from build123d import *

# Parameters (mm, degrees)
SKETCH1_W                     = 113.95
SKETCH1_H                     = 50
BOSS_EXTRUDE1_DEPTH           = 2
SKETCH2_W                     = 8
SKETCH2_H                     = 50
BOSS_EXTRUDE2_DEPTH           = 3
SKETCH3_W                     = 2
SKETCH3_H                     = 50
BOSS_EXTRUDE3_DEPTH           = 4
SKETCH7_W                     = 6
SKETCH7_H                     = 8
BOSS_EXTRUDE5_DEPTH           = 8
FILLET1_RADIUS                = 3
FILLET1_LENGTH                = 8
SKETCH10_R                    = 1.525
CUT_EXTRUDE2_DEPTH            = 2
LPATTERN2_COUNT               = 2
LPATTERN2_PITCH               = 20
FILLET1_OF_LPATTERN2_2_RADIUS = 3
FILLET1_OF_LPATTERN2_2_LENGTH = 8
FILLET2_R                     = 3
FILLET3_R                     = 3
FILLET4_START                 = -25
FILLET4_DEPTH                 = 20
FILLET4_START_2               = 3
FILLET4_2_DEPTH               = 12
FILLET4_START_3               = -19.719
FILLET4_3_DEPTH               = 44.719
FILLET4_START_4               = 23
FILLET4_4_DEPTH               = 2
FILLET5_R                     = 3


with BuildPart() as part:
    # Sketch1 → Boss-Extrude1 (new body)
    with BuildSketch(Plane(origin=(0, 0, 0), x_dir=(1, 0, 0), z_dir=(0, 1, 0))):
        Rectangle(SKETCH1_W, SKETCH1_H)
    extrude(amount=BOSS_EXTRUDE1_DEPTH)

    # Sketch2 → Boss-Extrude2 (add)
    with BuildSketch(Plane(origin=(0, 2, 0), x_dir=(1, 0, 0), z_dir=(0, 1, 0))):
        with Locations((-52.975, 0)):
            Rectangle(SKETCH2_W, SKETCH2_H)
    extrude(amount=BOSS_EXTRUDE2_DEPTH)

    # Sketch3 → Boss-Extrude3 (add)
    with BuildSketch(Plane(origin=(0, 2, 0), x_dir=(1, 0, 0), z_dir=(0, 1, 0))):
        with Locations((55.975, 0)):
            Rectangle(SKETCH3_W, SKETCH3_H)
    extrude(amount=BOSS_EXTRUDE3_DEPTH)

    # Sketch7 → Boss-Extrude5 (add)
    with BuildSketch(Plane(origin=(0, 5, 0), x_dir=(1, 0, 0), z_dir=(0, 1, 0))):
        with Locations((-53.975, 1)):
            Rectangle(SKETCH7_W, SKETCH7_H)
    boss_extrude5 = extrude(amount=BOSS_EXTRUDE5_DEPTH)

    # Fillet1: full round fillet: the end face becomes a half cylinder, R = half its width
    fillet1_face = Plane((-53.975, 13, -1), x_dir=(0, 0, 1), z_dir=(0, 1, 0))  # on the end face: x along it, z out of the body
    fillet1_slab = fillet1_face.offset(-FILLET1_RADIUS / 2) * Box(FILLET1_LENGTH, 2 * FILLET1_RADIUS, FILLET1_RADIUS, mode=Mode.PRIVATE)  # the body's end, R deep
    fillet1_round = Plane((-53.975, 10, -1), x_dir=(0, 1, 0), z_dir=(0, 0, 1)) * Cylinder(FILLET1_RADIUS, FILLET1_LENGTH, mode=Mode.PRIVATE)  # its axis R under the face
    add(fillet1_slab - fillet1_round, mode=Mode.SUBTRACT)

    # Sketch10 → Cut-Extrude2 (cut)
    with BuildSketch(Plane(origin=(0, 0, -5), x_dir=(-1, 0, 0), z_dir=(0, 0, -1))):
        with Locations((53.975, 10)):
            Circle(SKETCH10_R)
    cut_extrude2 = extrude(amount=-CUT_EXTRUDE2_DEPTH, mode=Mode.SUBTRACT)

    # LPattern2: Boss-Extrude5, Cut-Extrude2 ×2
    with Locations(*[(0, 0, i * LPATTERN2_PITCH) for i in range(1, LPATTERN2_COUNT)]):
        add(boss_extrude5)
        add(cut_extrude2, mode=Mode.SUBTRACT)

    # Fillet1 of LPattern2 2: full round fillet: the end face becomes a half cylinder, R = half its width
    fillet1_of_lpattern2_2_face = Plane((-53.975, 13, 19), x_dir=(0, 0, 1), z_dir=(0, 1, 0))  # on the end face: x along it, z out of the body
    fillet1_of_lpattern2_2_slab = fillet1_of_lpattern2_2_face.offset(-FILLET1_OF_LPATTERN2_2_RADIUS / 2) * Box(FILLET1_OF_LPATTERN2_2_LENGTH, 2 * FILLET1_OF_LPATTERN2_2_RADIUS, FILLET1_OF_LPATTERN2_2_RADIUS, mode=Mode.PRIVATE)  # the body's end, R deep
    fillet1_of_lpattern2_2_round = Plane((-53.975, 10, 19), x_dir=(0, 1, 0), z_dir=(0, 0, 1)) * Cylinder(FILLET1_OF_LPATTERN2_2_RADIUS, FILLET1_OF_LPATTERN2_2_LENGTH, mode=Mode.PRIVATE)  # its axis R under the face
    add(fillet1_of_lpattern2_2_slab - fillet1_of_lpattern2_2_round, mode=Mode.SUBTRACT)

    # Fillet2
    # the kernel refuses this fillet: 3 mm, written as the material it takes off along each edge
    with BuildSketch(Plane(origin=(-64.475, 0, -25), x_dir=(0, 1, 0), z_dir=(1, 0, 0))) as fillet2_piece_1:
        with BuildLine():
            CenterArc((FILLET2_R, FILLET2_R), FILLET2_R, 180, 90)
            Line((0, FILLET2_R), (0, 0))
            Line((0, 0), (FILLET2_R, 0))
        make_face()
    extrude(amount=128.95, mode=Mode.SUBTRACT)
    with BuildSketch(Plane(origin=(-56.975, 0, 32.5), x_dir=(1, 0, 0), z_dir=(0, 0, -1)), Plane(origin=(56.975, 0, -32.5), x_dir=(-1, 0, 0), z_dir=(0, 0, 1))) as fillet2_piece_2:
        with BuildLine():
            CenterArc((FILLET2_R, -FILLET2_R), FILLET2_R, 90, 90)
            Line((0, -FILLET2_R), (0, 0))
            Line((0, 0), (FILLET2_R, 0))
        make_face()
    extrude(amount=65, mode=Mode.SUBTRACT)
    with BuildSketch(Plane(origin=(64.475, 0, 25), x_dir=(0, 0, -1), z_dir=(-1, 0, 0))) as fillet2_piece_3:
        with BuildLine():
            CenterArc((FILLET2_R, -FILLET2_R), FILLET2_R, 90, 90)
            Line((0, -FILLET2_R), (0, 0))
            Line((0, 0), (FILLET2_R, 0))
        make_face()
    extrude(amount=128.95, mode=Mode.SUBTRACT)

    # Fillet3
    fillet3_edges = [part.edges().sort_by_distance(p)[0] for p in [
        (-48.975, 2, 0),
        (54.975, 2, 0),
    ]]
    fillet(fillet3_edges, radius=FILLET3_R - 0.0001)  # a hair under: the kernel refuses the full size

    # Fillet4: read off the stored shape, not the designer's step
    # Fillet4 outline → Fillet4 (cut)
    with BuildSketch(Plane.XY.offset(FILLET4_START)):
        with BuildLine():
            ThreePointArc((-51.171152423, 5), (-49.671152423, 4.598076211), (-48.573076211, 3.5))
            ThreePointArc((-48.573076211, 3.5), (-48.872777479, 4.223542864), (-48.975, 5))
            Line((-48.975, 5), (-51.171152423, 5))
        make_face()
        with BuildLine():
            ThreePointArc((-56.975, 3), (-55.878623683, 4.449489743), (-54.146572875, 5))
            Line((-54.146572875, 5), (-56.975, 5))
            Line((-56.975, 5), (-56.975, 3))
        make_face()
    extrude(amount=FILLET4_DEPTH, mode=Mode.SUBTRACT)

    # Fillet4 2 outline → Fillet4 2 (cut)
    with BuildSketch(Plane.XY.offset(FILLET4_START_2)):
        with BuildLine():
            Line((-53.975, 5), (-56.975, 5))
            Line((-56.975, 5), (-56.975, 3))
            ThreePointArc((-56.975, 3), (-56.964491568, 2.749121219), (-56.933039892, 2.5))
            ThreePointArc((-56.933039892, 2.5), (-55.911491673, 4.291287847), (-53.975, 5))
        make_face()
        with BuildLine():
            ThreePointArc((-51.171152423, 5), (-49.671152423, 4.598076211), (-48.573076211, 3.5))
            ThreePointArc((-48.573076211, 3.5), (-48.872777479, 4.223542864), (-48.975, 5))
            Line((-48.975, 5), (-51.171152423, 5))
        make_face()
    extrude(amount=FILLET4_2_DEPTH, mode=Mode.SUBTRACT)

    # Fillet4 3 outline → Fillet4 3 (cut)
    with BuildSketch(Plane.XY.offset(FILLET4_START_3)):
        with BuildLine():
            Line((-50.975, 5), (-50.975, 4.993580503))
            ThreePointArc((-50.975, 4.993580503), (-49.58697311, 4.547621617), (-48.573076211, 3.5))
            ThreePointArc((-48.573076211, 3.5), (-48.872777479, 4.223542864), (-48.975, 5))
            Line((-48.975, 5), (-50.975, 5))
        make_face()
    extrude(amount=FILLET4_3_DEPTH, mode=Mode.SUBTRACT)

    # Fillet4 4 outline → Fillet4 4 (cut)
    with BuildSketch(Plane.XY.offset(FILLET4_START_4)):
        with BuildLine():
            Line((-50.975, 5), (-51.171152423, 5))
            ThreePointArc((-51.171152423, 5), (-51.073023703, 4.998394696), (-50.975, 4.993580503))
            Line((-50.975, 4.993580503), (-50.975, 5))
        make_face()
        with BuildLine():
            ThreePointArc((-56.975, 3), (-55.878623683, 4.449489743), (-54.146572875, 5))
            Line((-54.146572875, 5), (-56.975, 5))
            Line((-56.975, 5), (-56.975, 3))
        make_face()
    extrude(amount=FILLET4_4_DEPTH, mode=Mode.SUBTRACT)

    # Fillet5
    # the kernel refuses this fillet: 3 mm, written as the material it takes off along each edge
    with BuildSketch(Plane(origin=(56.975, 6, 32.071067812), x_dir=(0, -1, 0), z_dir=(0, 0, -1))) as fillet5_piece_1:
        with BuildLine():
            CenterArc((2.828427125, 3), FILLET5_R, 199.471220634, 70.528779366)
            Line((0, 2), (-0.056568542, 1.98))
            ThreePointArc((-0.056568542, 1.98), (-0.06, 1), (-0.06, 0))
            Line((-0.06, 0), (0, -0.06))
            Line((0, -0.06), (2.828427125, -0.06))
            Line((2.828427125, -0.06), (2.828427125, 0))
        make_face()
    extrude(amount=64.142135624, mode=Mode.SUBTRACT)


solid = part.part
Here's how the part is built. I have some questions about the finished solid (model axes, mm). A direction names the side the tool comes from. Coordinates: 2 decimals unless noted, no trailing zeros. Order: outer loops, then holes, each group sorted by start corner. A loop starts at its lowest first (then second) coordinate and runs counter-clockwise, first axis right, second up. Notation, with made-up numbers: (-8.5, 79) - (-2.5, 79) arc R23 ccw to (-2.5, 114) - close; hole circle Ø4 at (88.5, -32). An arc over 180 degrees is marked (long way). Use CSV: the item, a comma, the result in double quotes. Start each with the question number.
1. If we mould it in two halves opening along X, with no side actions, what happens to faces 6 (the face through (-54, 8, 15)), 7 (the face through (-47.46, 2.394, -0.35)), 8 (the face through (-56.975, 6, 19))? For each: +X half, -X half, draft (parallel to the pull), parting line (faces both ways), or undercut.
2. Suppose I cut it at B-B on x = 46. List the corners of the cut face in (y, z) for me, then the cut area to 4 significant figures.
3. Suppose I cut it at A-A on z = 11.5. List the corners of the cut face in (x, y) for me (3 decimals).
4. Please list where these lines run through material, in increasing order: line 1 (Y direction, x = -34.5, z = -20); line 2 (X direction, y = 2.5, z = 22.5); line 3 (X direction, y = 4.75, z = 9). Write a range as from..to.
5. I'm going to push flat-ended pins straight in: pin 1 (0.6 mm diameter, centred on x = -53, z = 24, fed in from +Y); pin 2 (3.5 mm diameter, centred on x = -53.975, y = 10, fed in from -Z); pin 3 (5 mm diameter, centred on x = -53.975, y = 10, fed in from +Z); pin 4 (1 mm diameter, centred on y = 8, z = -15.5, fed in from -X). Where does each tip first touch, or does it pass through?
6. For faces 1 (the face through (-50.975, 8, 19)), 2 (the face through (-54, 8, -5)), 3 (the face through (-53, 5, 24)), 4 (the face through (-53, 5, 9)), 5 (the face through (-53.776, 11.512, -4.014)), which set-ups out of +Z, -Z, +X, -X, +Y, -Y let a thin tool reach every point of the face, with its end or its side?
7. Suppose I cut it at C-C on z = 18.5. List the corners of the cut face in (x, y) for me (3 decimals).
Output:
1,face 6,"draft"
1,face 7,"undercut"
1,face 8,"-X half"
2,outline,"(0, -22) arc R3 ccw to (2, -24.83) - (2, 24.83) arc R3 ccw to (0, 22) - close"
2,area,"96.25 mm2"
3,outline,"(-56.933, 2.5) arc R3 ccw to (-53.975, 0) - (53.975, 0) arc R3 ccw to (56.975, 3) - (56.975, 3.172) arc R3 ccw to (54.975, 6) - (54.975, 5) arc R3 cw to (51.975, 2) - (-45.975, 2) arc R3 cw to (-48.578, 3.509) arc R3 ccw to (-51.171, 5) - (-53.975, 5) arc R3 ccw to start"
4,line 1,"y = 0..2"
4,line 2,"x = -56.93..-47.63, 53.63..56.93"
4,line 3,"x = -55.17..-49.97, 54.96..56.53"
5,pin 1,"stops at y = 5"
5,pin 2,"stops at z = -5"
5,pin 3,"stops at z = 23"
5,pin 4,"passes through"
6,face 1,"+Z, -Z, +Y"
6,face 2,"-Z, -X, +Y"
6,face 3,"+Z, -X, +Y"
6,face 4,"-X, +Y"
6,face 5,"-Z"
7,outline,"(-56.975, 3) arc R3 ccw to (-53.975, 0) - (53.975, 0) arc R3 ccw to (56.975, 3) - (56.975, 3.172) arc R3 ccw to (54.975, 6) - (54.975, 5) arc R3 cw to (51.975, 2) - (-45.975, 2) arc R3 cw to (-48.578, 3.509) arc R3 ccw to (-50.975, 4.994) - (-50.975, 10) arc R3 ccw to (-56.975, 10) - close"
